Autodesk Inventor part; units mm, degrees
ref_plane "YZ Plane" through (0, 0, 0) normal (1, 0, 0) x (0, 1, 0)
ref_plane "XZ Plane" through (0, 0, 0) normal (0, 1, 0) x (-1, 0, 0)
ref_plane "XY Plane" through (0, 0, 0) normal (0, 0, 1) x (1, 0, 0)
sketch "Sketch1" plane through (0, 0, 0) normal (0, 0, 1) x (1, 0, 0)
  line L0 (77.9423, 0) -> (38.9711, -67.5)
  line L1 (38.9711, -67.5) -> (-38.9711, -67.5)
  line L2 (-38.9711, -67.5) -> (-77.9423, 0)
  line L3 (-77.9423, 0) -> (-38.9711, 67.5)
  line L4 (-38.9711, 67.5) -> (38.9711, 67.5)
  line L5 (38.9711, 67.5) -> (77.9423, 0)
  circle A0 centre (0, 0) radius 12.5
  circle A1 centre (54, 0) radius 2.5
  circle A2 centre (46.7654, 27) radius 2.5
  circle A3 centre (27, 46.7654) radius 2.5
  circle A4 centre (0, 54) radius 2.5
  circle A5 centre (-27, 46.7654) radius 2.5
  circle A6 centre (-46.7654, 27) radius 2.5
  circle A7 centre (-54, 0) radius 2.5
  circle A8 centre (-46.7654, -27) radius 2.5
  circle A9 centre (-27, -46.7654) radius 2.5
  circle A10 centre (0, -54) radius 2.5
  circle A11 centre (27, -46.7654) radius 2.5
  circle A12 centre (46.7654, -27) radius 2.5
  dimension "d0" = 135
  dimension "d1" = 25
  dimension "d2" = 54
  dimension "d3" = 5
  dimension "d6" = 360
extrude "Extrusion1" add sketch "Sketch1" along normal blind 7
sketch "Sketch5" plane through (0, 0, 7) normal (0, 0, 1) x (1, 0, 0)
  circle A0 centre (0, 0) radius 12.5
  circle A1 centre (46.7654, -27) radius 2.5
  circle A2 centre (27, -46.7654) radius 2.5
  circle A3 centre (-27, -46.7654) radius 2.5
  circle A4 centre (-46.7654, -27) radius 2.5
  circle A5 centre (-54, 0) radius 2.5
  circle A6 centre (-46.7654, 27) radius 2.5
  circle A7 centre (-27, 46.7654) radius 2.5
  circle A8 centre (27, 46.7654) radius 2.5
  circle A9 centre (46.7654, 27) radius 2.5
  circle A10 centre (54, 0) radius 2.5
  line L0 (38.9711, -67.5) -> (77.9423, 0)
  line L1 (77.9423, 0) -> (38.9711, 67.5)
  line L2 (38.9711, 67.5) -> (-38.9711, 67.5)
  line L3 (-38.9711, 67.5) -> (-77.9423, 0)
  line L4 (-77.9423, 0) -> (-38.9711, -67.5)
  line L5 (-38.9711, -67.5) -> (38.9711, -67.5)
  line L6 (-68.1273, 0) -> (-34.0637, 59)
  line L7 (-34.0637, 59) -> (34.0637, 59)
  line L8 (34.0637, 59) -> (68.1273, 0)
  line L9 (68.1273, 0) -> (34.0637, -59)
  line L10 (34.0637, -59) -> (-34.0637, -59)
  line L11 (-34.0637, -59) -> (-68.1273, 0)
  dimension "d30" = 118
extrude "Extrusion5" cut sketch "Sketch5" against normal through all contours L5 L4 L3 L2 L1 L0
sketch "Sketch6" plane through (0, 0, 7) normal (0, 0, 1) x (1, 0, 0)
  circle A0 centre (0, 52) radius 2.5
  circle A1 centre (-13.4586, 50.2281) radius 2.5
  circle A2 centre (-26, 45.0333) radius 2.5
  circle A3 centre (-36.7696, 36.7696) radius 2.5
  circle A4 centre (-45.0333, 26) radius 2.5
  circle A5 centre (-50.2281, 13.4586) radius 2.5
  circle A6 centre (-52, 0) radius 2.5
  circle A7 centre (-50.2281, -13.4586) radius 2.5
  circle A8 centre (-45.0333, -26) radius 2.5
  circle A9 centre (-36.7696, -36.7696) radius 2.5
  circle A10 centre (-26, -45.0333) radius 2.5
  circle A11 centre (-13.4586, -50.2281) radius 2.5
  circle A12 centre (0, -52) radius 2.5
  circle A13 centre (13.4586, -50.2281) radius 2.5
  circle A14 centre (26, -45.0333) radius 2.5
  circle A15 centre (36.7696, -36.7696) radius 2.5
  circle A16 centre (45.0333, -26) radius 2.5
  circle A17 centre (50.2281, -13.4586) radius 2.5
  circle A18 centre (52, 0) radius 2.5
  circle A19 centre (50.2281, 13.4586) radius 2.5
  circle A20 centre (45.0333, 26) radius 2.5
  circle A21 centre (36.7696, 36.7696) radius 2.5
  circle A22 centre (26, 45.0333) radius 2.5
  circle A23 centre (13.4586, 50.2281) radius 2.5
  point P0 (0, 0)
  dimension "d35" = 5
  dimension "d38" = 360
  dimension "d40" = 52
extrude "Extrusion6" cut sketch "Sketch6" against normal through all contours A11 | A23
sketch "Sketch7" plane through (0, 0, 7) normal (0, 0, 1) x (1, 0, 0)
  circle A0 centre (13.4586, 50.2281) radius 2.5
  circle A1 centre (-13.4586, -50.2281) radius 2.5
  circle A2 centre (13.4586, 50.2281) radius 6.5
  circle A3 centre (-13.4586, -50.2281) radius 6.5
  point P0 (0, 0)
  dimension "d43" = 13
  dimension "d44" = 13
extrude "Extrusion7" cut sketch "Sketch7" against normal blind 5 contours A0 | A1 | A2 | A3
properties part number "AC04" material "ABS Plastic"
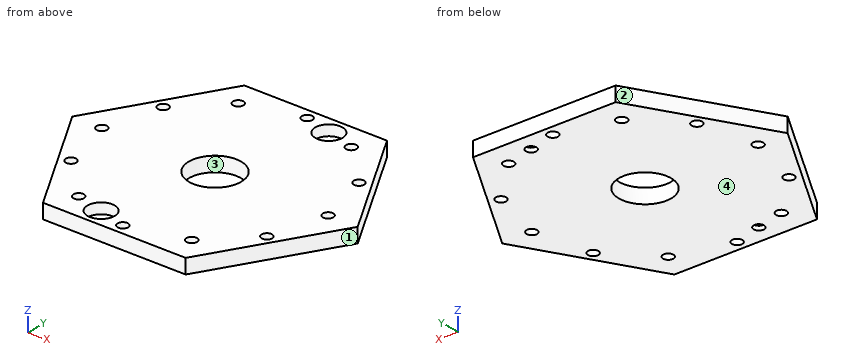
Check sheet for the modelled part. Datum: model origin and axes. Units: mm. Face numbers are marked on the shaded views. Round coordinates to 2 decimals unless told otherwise and drop trailing zeros. Loops run counter-clockwise (first coordinate to the right, second up) from the corner with the lowest first, then second, coordinate; pieces in that order, holes last. Notation, with made-up numbers: (29, -30.5) -> (37, -30.5) arc R22 ccw to (37, -18.5) -> close; hole circle Ø1 at (-22, 44.5). An arc over 180 degrees is marked (long way). Write item = value, one per line. Start each with the question number.
1) Thickness scan on probe 1 along Y at (x, z) = (27, 3); probe 2 along Y at (x, z) = (0, 6); probe 3 along X at (y, z) = (53.5, 5.75). Record the ranges inside material, lowest first.
2) Gauge pin test, flat ends, axial feed: pin 1 Ø1.5 at (y, z) = (-38, 4.5) entering from -X; pin 2 Ø1 at (y, z) = (-4.5, 5) entering from +X; pin 3 Ø1 at (x, z) = (-40, 5.5) entering from +Y. Record the tip position at first contact, or that the pin passes through.
3) Sectioned sample at C-C, the plane z = 4.25. State how many separate pieces and enclosed holes the cut face has, plus the area to 3 significant figures.
4) Sectioned sample at B-B, the plane y = -27. Record the cut outline in (x, z).
5) Release check for a two-part mould opening along Y. For the marked faces 1, 2, 3 and 4 record: released by +Y, released by -Y, zero draft, split by the parting line, or undercut.
6) Sectioned sample at A-A, the plane x = 0. Record the cut outline in (y, z).
7) Sectioned sample at D-D, the plane x = -54. Record the cut outline in (y, z), plus the area to 3 significant figures.
Results are:
q1.probe_1 = -59 to -49.27, -44.27 to 44.27, 49.27 to 59
q1.probe_2 = -59 to -56.5, -51.5 to -12.5, 12.5 to 51.5, 56.5 to 59
q1.probe_3 = -37.24 to -2.45, 2.45 to 7.84, 19.08 to 37.24
q2.pin_1 = -46.62
q2.pin_2 = 65.82
q2.pin_3 = 49.58
q3.separate_pieces = 1
q3.enclosed_holes = 15
q3.area = 11,100 mm^2
q4.outline = (-52.54, 0) -> (-49.27, 0) -> (-49.27, 7) -> (-52.54, 7) -> close; (-44.27, 0) -> (44.27, 0) -> (44.27, 7) -> (-44.27, 7) -> close; (49.27, 0) -> (52.54, 0) -> (52.54, 7) -> (49.27, 7) -> close
q5.face_1 = released by -Y
q5.face_2 = released by +Y
q5.face_3 = undercut
q5.face_4 = zero draft
q6.outline = (-59, 0) -> (-56.5, 0) -> (-56.5, 7) -> (-59, 7) -> close; (-51.5, 0) -> (-12.5, 0) -> (-12.5, 7) -> (-51.5, 7) -> close; (12.5, 0) -> (51.5, 0) -> (51.5, 7) -> (12.5, 7) -> close; (56.5, 0) -> (59, 0) -> (59, 7) -> (56.5, 7) -> close
q7.outline = (-24.47, 0) -> (-2.5, 0) -> (-2.5, 7) -> (-24.47, 7) -> close; (2.5, 0) -> (24.47, 0) -> (24.47, 7) -> (2.5, 7) -> close
q7.area = 308 mm^2
